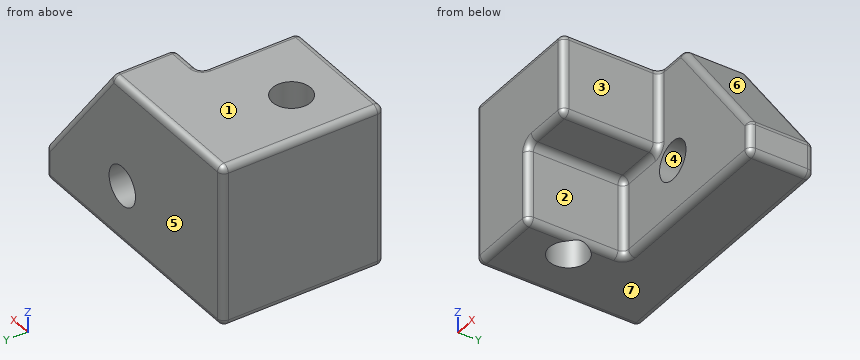
```python
from build123d import *

# Parameters (mm, degrees)
F0_W     = 203.2
F0_H     = 127
F1_DEPTH = 127
F3_DEPTH = 76.2
F4_SIZE2 = 101.6
F4_SIZE  = 76.2
F5_R     = 5.08
F6_R     = 15.24
F7_DEPTH = 50.8
F8_R     = 14.8914565461
F9_DEPTH = 127


with BuildPart() as f1:
    # F0 (on Front) → F1 (new body)
    with BuildSketch(Plane.XZ):
        with Locations((1.736553802, 1.4607831836)):
            Rectangle(F0_W, F0_H)
    extrude(amount=F1_DEPTH)

    # F2 (on face) → F3 (cut)
    with BuildSketch(Plane.XZ.offset(127)):
        Polygon((0, 64.9607831836), (0, 0), (-40.8341363072, 0), (-40.8341363072, -62.0392168164), (103.336553802, -62.0392168164), (103.336553802, 64.9607831836), align=None)
    extrude(amount=-F3_DEPTH, mode=Mode.SUBTRACT)

    # F4
    f4_edges = [f1.edges().sort_by_distance(p)[0] for p in [
        (103.336554, -25.4, 64.960783),
    ]]
    f4_side = f1.faces().sort_by_distance((-20.189124, -52.346525, 64.960783))[0]
    chamfer(f4_edges, length=F4_SIZE, length2=F4_SIZE2, reference=f4_side)

    # F5
    f5_edges = [f1.edges().sort_by_distance(p)[0] for p in [
        (-99.863446, -63.5, 64.960783),
        (-49.931723, -127, 64.960783),
        (0, -88.9, 64.960783),
        (27.136554, -25.4, 64.960783),
        (13.568277, -50.8, 64.960783),
        (65.236554, -50.8, 14.160783),
        (0, -50.8, 32.480392),
        (0, -127, 32.480392),
        (31.251209, -50.8, -62.039217),
        (103.336554, -50.8, -49.339217),
        (103.336554, -25.4, -36.639217),
        (103.336554, -25.4, -62.039217),
        (103.336554, 0, -49.339217),
        (65.236554, 0, 14.160783),
        (-20.417068, -127, 0),
        (-40.834136, -127, -31.019608),
        (-40.834136, -88.9, -62.039217),
        (-40.834136, -50.8, -31.019608),
        (0, -88.9, 0),
        (-40.834136, -88.9, 0),
        (-99.863446, -63.5, -62.039217),
        (-70.348791, -127, -62.039217),
        (1.736554, 0, -62.039217),
        (-99.863446, -127, 1.460783),
        (-99.863446, 0, 1.460783),
        (-36.363446, 0, 64.960783),
        (-20.417068, -50.8, 0),
    ]]
    fillet(f5_edges, radius=F5_R)

    # F6 (on face) → F7 (cut, through all)
    with BuildSketch(Plane.XZ.offset(50.8)):
        with Locations((15.0458636928, -16.3192168164)):
            Circle(F6_R)
    extrude(amount=-F7_DEPTH, mode=Mode.SUBTRACT)

    # F8 (on face) → F9 (cut, through all)
    with BuildSketch(Plane.XY.offset(64.9607831836)):
        with Locations((-56.683446198, -83.82)):
            Circle(F8_R)
    extrude(amount=-F9_DEPTH, mode=Mode.SUBTRACT)


solid = f1.part
```
Source: CAD feature listing. Evaluate the final solid. Frame: model axes, mm. Face numbers are marked on the shaded views. A direction names the side the tool comes from. Give positions to 0.01 mm unless a question says otherwise; leave off trailing zeros. Write each loop counter-clockwise with the first axis right and the second up, starting at its lowest first coordinate (ties: lowest second). Pieces come first, ordered by that corner, then holes.
1. Material intervals for line 1 along X through (y, z) = (-83.82, -6.5); line 2 along Y through (x, z) = (57, -10); line 3 along X through (y, z) = (-67.5, -15.5), sorted ascending.
2. Section query A-A (z = -42). Return the cut outline in (x, y).
3. Pull-direction query (Z, two-part tool) for the marked faces 4, 5, 6 and 7; classes: +Z half, -Z half, draft (parallel to the pull), parting line (faces both ways), or undercut.
4. First-contact query: pin 1 (8 mm diameter, centred on x = 26, z = -24, fed in from -Y); pin 2 (10 mm diameter, centred on x = 44, z = 44, fed in from -Y); pin 3 (12 mm diameter, centred on y = -81, z = -46.5, fed in from +X). Flat tips, straight axial feed; report the tip coordinate or a pass-through.
5. Section query B-B (y = -78). Return the cut outline in (x, z), then the cut area to 3 significant figures.
6. Access query for the marked faces 1, 2 and 3. Directions: +Z, -Z, +X, -X, +Y, -Y. A direction counts if a zero-diameter tool reaches every point of the face in a straight line with its end or side. Return the directions, or none.
7. Section query C-C (y = -63.5). Return the cut outline in (x, z), then the cut area to 3 significant figures.
8. Section query D-D (y = -12). Return the cut outline in (x, z), then the cut area to 3 significant figures.
Output values:
1. line 1: x = -99.86 to -71.57, -41.79 to -40.83
1. line 2: y = -50.8 to 0
1. line 3: x = -99.86 to -40.83
2. outline: (-99.86, -121.92) arc R5.08 ccw to (-94.78, -127) - (-45.91, -127) arc R5.08 ccw to (-40.83, -121.92) - (-40.83, -55.88) arc R5.08 cw to (-35.75, -50.8) - (98.26, -50.8) arc R5.08 ccw to (103.34, -45.72) - (103.34, -5.08) arc R5.08 ccw to (98.26, 0) - (-94.78, 0) arc R5.08 ccw to (-99.86, -5.08) - close; hole circle Ø29.78 at (-56.68, -83.82)
3. face 4: undercut
3. face 5: draft
3. face 6: +Z half
3. face 7: -Z half
4. pin 1: stops at y = -50.8
4. pin 2: stops at y = -50.7
4. pin 3: stops at x = -40.83
5. outline: (-99.86, -56.96) arc R5.08 ccw to (-94.78, -62.04) - (-70.39, -62.04) - (-70.39, 64.96) - (-94.78, 64.96) arc R5.08 ccw to (-99.86, 59.88) - close; (-42.98, -61.1) arc R5.08 ccw to (-40.83, -56.96) - (-40.83, -5.08) arc R5.08 cw to (-35.75, 0) - (-5.08, 0) arc R5.08 ccw to (0, 5.08) - (0, 59.88) arc R5.08 ccw to (-5.08, 64.96) - (-42.98, 64.96) - close
5. area: 6,650 mm2
6. face 1: +Z, +X, -X, +Y, -Y
6. face 2: -Z, +X, -Y
6. face 3: +Z, -Z, +X, -Y
7. outline: (-99.86, -56.96) arc R5.08 ccw to (-94.78, -62.04) - (-45.91, -62.04) arc R5.08 ccw to (-40.83, -56.96) - (-40.83, -5.08) arc R5.08 cw to (-35.75, 0) - (-5.08, 0) arc R5.08 ccw to (0, 5.08) - (0, 59.88) arc R5.08 ccw to (-5.08, 64.96) - (-94.78, 64.96) arc R5.08 ccw to (-99.86, 59.88) - close
7. area: 10,100 mm2
8. outline: (-99.86, -56.96) arc R5.08 ccw to (-94.78, -62.04) - (98.26, -62.04) arc R5.08 ccw to (103.34, -56.96) - (103.34, -38.33) arc R5.08 ccw to (102.32, -35.28) - (28.66, 62.93) arc R5.08 ccw to (24.6, 64.96) - (-94.78, 64.96) arc R5.08 ccw to (-99.86, 59.88) - close; hole circle Ø30.48 at (15.05, -16.32)
8. area: 21,200 mm2
